```python
from build123d import *

# Parameters (mm, degrees)
SKETCH_2_W          = 10
SKETCH_2_H          = 4
CUT_EXTRUDE_1_DEPTH = 27


with BuildPart() as part:
    # 草圖1 → 旋轉1 (revolve)
    with BuildSketch(Plane.XY):
        Polygon((30, -13), (30, -3), (12.5, -3), (12.5, -13), (8, -13), (8, 13), (12.5, 13), (12.5, 3), (30, 3), (30, 13), (40, 13), (40, 10), (32, 7.088238126), (32, 4.411761874), (40, 1.5), (40, -1.5), (32, -4.411761874), (32, -7.088238126), (40, -10), (40, -13), align=None)
    revolve(axis=Axis((0, 0, 0), (0, 1, 0)))

    # 草圖2 → 除料-伸長1 (cut, through all)
    with BuildSketch(Plane(origin=(0, 13, 0), x_dir=(1, 0, 0), z_dir=(0, 1, 0))):
        with Locations((5, 0)):
            Rectangle(SKETCH_2_W, SKETCH_2_H)
    extrude(amount=-CUT_EXTRUDE_1_DEPTH, mode=Mode.SUBTRACT)


solid = part.part
```
Part model, mm, in its own coordinate system. A direction names the side the tool comes from. Round coordinates to 2 decimals unless told otherwise and drop trailing zeros. Loops run counter-clockwise (first coordinate to the right, second up) from the corner with the lowest first, then second, coordinate; pieces in that order, holes last. Notation, with made-up numbers: (40, 54.5) -> (89, 54.5) arc R34 cw to (89, 89.5) -> close; hole circle Ø9 at (15.5, 24.25). An arc over 180 degrees is marked (long way). Use a Markdown table: item, result.
1) Cut at B-B, the plane y = -0.5. List the corners of the cut face in (x, z), and give its area (3 significant figures).
The answers:
| item | result |
|---|---|
| outline | circle Ø80 at (0, 0); hole (7.75, -2) -> (10, -2) -> (10, 2) -> (7.75, 2) arc R8 ccw (long way) to start |
| area | 4,820 mm2 |
2) Pull direction Z, two halves, no side cores. Call faces 6 (the flat face through (-6, 13, -30)), 7 (the cylindrical face through (-8.67, -11.52, 39.05)), 8 (the flat face through (9, 0, -2)): pulls with the +Z half, pulls with the -Z half, needs draft (parallel to the pull), parting line crosses it, or undercut.
The answers:
| item | result |
|---|---|
| face 6 | needs draft |
| face 7 | parting line crosses it |
| face 8 | undercut |
3) Probe line 1 (X direction, y = -6, z = 0); line 2 (X direction, y = -6.5, z = -6); line 3 (Z direction, x = 0, y = 6.25). List the from-to ranges inside material, lowest first. Write a range as [from, to].
The answers:
| item | result |
|---|---|
| line 1 | x = [-32, -30], [-12.5, -8], [10, 12.5], [30, 32] |
| line 2 | x = [-31.43, -29.39], [-10.97, -5.29], [5.29, 10.97], [29.39, 31.43] |
| line 3 | z = [-32, -30], [-12.5, -8], [8, 12.5], [30, 32] |
4) Cut at A-A, the plane y = 5.75. List the corners of the cut face in (x, z).
The answers:
| item | result |
|---|---|
| outline | circle Ø64 at (0, 0); circle Ø25 at (0, 0); hole circle Ø60 at (0, 0); hole (7.75, -2) -> (10, -2) -> (10, 2) -> (7.75, 2) arc R8 ccw (long way) to start |
5) Tool access for faces 1 (the cylindrical face through (-6.94, 5.73, 31.24)), 2 (the cylindrical face through (11.923, 7.93, -3.755)), 3 (the cylindrical face through (11.923, -8.07, -3.755)), 4 (the flat face through (6, -13, -30)), 5 (the cylindrical face through (-8.67, 11.48, 39.05)): list every direction of +Z, -Z, +X, -X, +Y, -Y with a clear straight run to the whole face (end or side of a thin tool).
The answers:
| item | result |
|---|---|
| face 1 | none |
| face 2 | +Y |
| face 3 | -Y |
| face 4 | +Z, -Z, +X, -X, -Y |
| face 5 | +Y, -Y |
6) Drop flat-ended pins along their axis: pin 1 Ø1.1 at (x, y) = (8.5, -5) entering from +Z; pin 2 Ø9.5 at (x, z) = (0, 0) entering from -Y; pin 3 Ø2 at (x, z) = (16, -18.5) entering from +Y; pin 4 Ø10 at (x, y) = (3.5, -7) entering from -Z. Give the stop position or say it passes through.
The answers:
| item | result |
|---|---|
| pin 1 | stops at z = 31 |
| pin 2 | passes through |
| pin 3 | stops at y = 3 |
| pin 4 | stops at z = -40 |
7) Cut at C-C, the plane z = 33. State how many separate pieces and enclosed holes the cut face has, and give its area (3 significant figures).
The answers:
| item | result |
|---|---|
| separate pieces | 3 |
| enclosed holes | 0 |
| area | 708 mm2 |
